```python
from build123d import *

# Parameters (mm, degrees)
BOSS_EXTRUDE1_DEPTH      = 5
BOSS_EXTRUDE2_DEPTH      = 4
SKETCH3_W                = 3
SKETCH3_H                = 52.6
BOSS_EXTRUDE3_DEPTH      = 7
SKETCH4_R                = 2.5
BOSS_EXTRUDE4_DEPTH      = 5.5
SKETCH5_R                = 3.7
CUT_EXTRUDE2_DEPTH       = 1.6
CUT_EXTRUDE4_DEPTH       = 1.6
SKETCH7_R                = 2.5
CUT_EXTRUDE6_DEPTH       = 1.6
SKETCH8_R                = 1.5
CUT_EXTRUDE8_DEPTH       = 4
M2_CLEARANCE_HOLE1_D     = 2.4
M2_CLEARANCE_HOLE1_DEPTH = 5
M2_CLEARANCE_HOLE1_TIP   = 0.721032743
M2_CLEARANCE_HOLE2_D     = 2.4
M2_CLEARANCE_HOLE2_DEPTH = 5
M2_CLEARANCE_HOLE2_TIP   = 0.721032743
M2_CLEARANCE_HOLE3_D     = 2.4
M2_CLEARANCE_HOLE3_DEPTH = 35
M2_CLEARANCE_HOLE4_D     = 2.4
M2_CLEARANCE_HOLE4_DEPTH = 35
M2_CLEARANCE_HOLE5_D     = 2.4
M2_CLEARANCE_HOLE5_DEPTH = 35
M2_CLEARANCE_HOLE6_D     = 2.4
M2_CLEARANCE_HOLE6_DEPTH = 35
FILLET1_R                = 2
SKETCH21_W               = 15
SKETCH21_H               = 7
CUT_EXTRUDE10_DEPTH      = 4
SKETCH22_W               = 8
SKETCH22_H               = 9
CUT_EXTRUDE11_DEPTH      = 2.5


with BuildPart() as part:
    # Sketch1 → Boss-Extrude1 (new body)
    with BuildSketch(Plane(origin=(0, 19.3, 0), x_dir=(1, 0, 0), z_dir=(0, 1, 0))):
        with BuildLine():
            Line((5.5, -7), (33.5, -7))
            Line((33.5, -7), (33.5, 7))
            Line((33.5, 7), (5.5, 7))
            ThreePointArc((5.5, 7), (-1.5, 0), (5.5, -7))
        make_face()
    extrude(amount=BOSS_EXTRUDE1_DEPTH)



with BuildPart() as body_2:
    # Sketch2 → Boss-Extrude2 (new body)
    with BuildSketch(Plane(origin=(0, -28.3, 0), x_dir=(1, 0, 0), z_dir=(0, 1, 0))):
        with BuildLine():
            Line((5.5, -7), (33.5, -7))
            Line((33.5, -7), (33.5, 7))
            Line((33.5, 7), (5.5, 7))
            ThreePointArc((5.5, 7), (-1.5, 0), (5.5, -7))
        make_face()
    extrude(amount=BOSS_EXTRUDE2_DEPTH)


with BuildPart() as part_1:
    add(part.part)

    add(body_2.part)  # Boss-Extrude3 merges body 2
    # Sketch3 → Boss-Extrude3 (add, symmetric)
    with BuildSketch(Plane.XY):
        with Locations((32, -2)):
            Rectangle(SKETCH3_W, SKETCH3_H)
    extrude(amount=BOSS_EXTRUDE3_DEPTH, both=True)

    # Sketch4 → Boss-Extrude4 (add)
    with BuildSketch(Plane(origin=(0, 24.3, 0), x_dir=(1, 0, 0), z_dir=(0, 1, 0))):
        with Locations(Location((5.5, 0, 0), (0, 0, 270))):
            Circle(SKETCH4_R)
    extrude(amount=BOSS_EXTRUDE4_DEPTH)

    # Sketch5 → Cut-Extrude2 (cut)
    with BuildSketch(Plane(origin=(0, 19.3, 0), x_dir=(1, 0, 0), z_dir=(0, 1, 0))):
        with Locations(Location((5.5, 0, 0), (0, 0, 270))):
            Circle(SKETCH5_R)
    extrude(amount=CUT_EXTRUDE2_DEPTH, mode=Mode.SUBTRACT)

    # Sketch6 → Cut-Extrude4 (cut)
    with BuildSketch(Plane(origin=(0, 19.3, 0), x_dir=(1, 0, 0), z_dir=(0, 1, 0))):
        with BuildLine():
            Line((5.5, -2.7), (20.7, -2.7))
            Line((20.7, -2.7), (20.7, 2.7))
            Line((20.7, 2.7), (5.5, 2.7))
            ThreePointArc((5.5, 2.7), (2.8, 0), (5.5, -2.7))
        make_face()
    extrude(amount=CUT_EXTRUDE4_DEPTH, mode=Mode.SUBTRACT)

    # Sketch7 → Cut-Extrude6 (cut)
    with BuildSketch(Plane(origin=(0, 20.9, 0), x_dir=(1, 0, 0), z_dir=(0, 1, 0))):
        with Locations(Location((5.5, 0, 0), (0, 0, 270))):
            Circle(SKETCH7_R)
    extrude(amount=CUT_EXTRUDE6_DEPTH, mode=Mode.SUBTRACT)

    # Sketch8 → Cut-Extrude8 (cut)
    with BuildSketch(Plane(origin=(0, -28.3, 0), x_dir=(1, 0, 0), z_dir=(0, 1, 0))):
        with Locations(Location((5.5, 0, 0), (0, 0, 270))):
            Circle(SKETCH8_R)
    extrude(amount=CUT_EXTRUDE8_DEPTH, mode=Mode.SUBTRACT)

    # M2 Clearance Hole1
    with Locations(Plane(origin=(0, 24.3, 0), x_dir=(1, 0, 0), z_dir=(0, 1, 0))):
        with Locations((15.5, 0)):
            Hole(M2_CLEARANCE_HOLE1_D / 2, depth=M2_CLEARANCE_HOLE1_DEPTH)
            with Locations((0, 0, -(M2_CLEARANCE_HOLE1_DEPTH + M2_CLEARANCE_HOLE1_TIP / 2))):  # 118° drill point
                Cone(0, M2_CLEARANCE_HOLE1_D / 2, M2_CLEARANCE_HOLE1_TIP, mode=Mode.SUBTRACT)

    # M2 Clearance Hole2
    with Locations(Plane(origin=(0, 24.3, 0), x_dir=(1, 0, 0), z_dir=(0, 1, 0))):
        with Locations((18.5, 0)):
            Hole(M2_CLEARANCE_HOLE2_D / 2, depth=M2_CLEARANCE_HOLE2_DEPTH)
            with Locations((0, 0, -(M2_CLEARANCE_HOLE2_DEPTH + M2_CLEARANCE_HOLE2_TIP / 2))):  # 118° drill point
                Cone(0, M2_CLEARANCE_HOLE2_D / 2, M2_CLEARANCE_HOLE2_TIP, mode=Mode.SUBTRACT)

    # M2 Clearance Hole3
    with Locations(Plane(origin=(33.5, 0, 0), x_dir=(0, 0, -1), z_dir=(1, 0, 0))):
        with Locations((4.5, -4.5)):
            Hole(M2_CLEARANCE_HOLE3_D / 2, depth=M2_CLEARANCE_HOLE3_DEPTH)

    # M2 Clearance Hole4
    with Locations(Plane(origin=(33.5, 0, 0), x_dir=(0, 0, -1), z_dir=(1, 0, 0))):
        with Locations((-4.5, -4.5)):
            Hole(M2_CLEARANCE_HOLE4_D / 2, depth=M2_CLEARANCE_HOLE4_DEPTH)

    # M2 Clearance Hole5
    with Locations(Plane(origin=(33.5, 0, 0), x_dir=(0, 0, -1), z_dir=(1, 0, 0))):
        with Locations((4.5, 4.5)):
            Hole(M2_CLEARANCE_HOLE5_D / 2, depth=M2_CLEARANCE_HOLE5_DEPTH)

    # M2 Clearance Hole6
    with Locations(Plane(origin=(33.5, 0, 0), x_dir=(0, 0, -1), z_dir=(1, 0, 0))):
        with Locations((-4.5, 4.5)):
            Hole(M2_CLEARANCE_HOLE6_D / 2, depth=M2_CLEARANCE_HOLE6_DEPTH)

    # Fillet1
    fillet1_edges = [part_1.edges().sort_by_distance(p)[0] for p in [
        (30.5, 19.3, 0),
        (30.5, -24.3, 0),
    ]]
    fillet(fillet1_edges, radius=FILLET1_R)

    # Sketch21 → Cut-Extrude10 (cut)
    with BuildSketch(Plane(origin=(0, -28.3, 0), x_dir=(1, 0, 0), z_dir=(0, 1, 0))):
        with Locations((19.5, 0)):
            Rectangle(SKETCH21_W, SKETCH21_H)
    extrude(amount=CUT_EXTRUDE10_DEPTH, mode=Mode.SUBTRACT)

    # Sketch22 → Cut-Extrude11 (cut)
    with BuildSketch(Plane(origin=(0, 24.3, 0), x_dir=(1, 0, 0), z_dir=(0, 1, 0))):
        with Locations((25, 0)):
            Rectangle(SKETCH22_W, SKETCH22_H)
    extrude(amount=-CUT_EXTRUDE11_DEPTH, mode=Mode.SUBTRACT)


solid = part_1.part
```
Source: CAD feature listing. Evaluate the final solid. Frame: model axes, mm. A direction names the side the tool comes from. Give positions to 0.01 mm unless a question says otherwise; leave off trailing zeros. Loops run counter-clockwise (first coordinate to the right, second up) from the corner with the lowest first, then second, coordinate; pieces in that order, holes last. Notation, with made-up numbers: (75.25, -32) -> (109.25, -32) arc R36 ccw to (109.25, 6) -> close; hole circle Ø1 at (-32.75, 53.5). An arc over 180 degrees is marked (long way). Put each result on its own line as item: value. Start each with the question number.
1) Cut plane B-B (y = -4.5). Return loops of the section in (x, z), then the cut area to 3 significant figures.
2) Draft query along X for faces 1 (the face through (1.8, 20.1, -0.1)), 2 (the face through (16, -28.3, 5)), 3 (the face through (29.9, -23.73, -0.1)). Return one class per face: released by +X, released by -X, zero draft, split by the parting line, or undercut.
3) Cut plane A-A (x = 10.5). Return loops of the section in (y, z).
4) Reachability of faces 4 (the face through (25, 21.8, 0)), 5 (the face through (17, 19.3, -3)), 6 (the face through (27, -26, 0)) from +Z, -Z, +X, -X, +Y, -Y: full face, straight path, thin tool, end or side. Return the list, or none.
5) Contact query for flat-ended pins moving along their axis: P1, Ø2.5, axis at x = 26, z = 1, coming from the +Y side; P2, Ø4, axis at x = 18.5, z = 3, coming from the +Y side; P3, Ø4, axis at y = 4.5, z = -4.5, coming from the -X side. Output: stop coordinate, or through.
6) Material intervals for probe 1 along Y at (x, z) = (31.5, -4.5); probe 2 along Z at (x, y) = (25.5, 24); probe 3 along Y at (x, z) = (28.5, -2.5), sorted ascending.
7) Cut plane C-C (x = 23.5). Return loops of the section in (y, z), then the cut area to 3 significant figures.
8) Cut plane D-D (x = 18.5). Return loops of the section in (y, z).
Results are:
1. outline: (30.5, -7) -> (33.5, -7) -> (33.5, -5.7) -> (30.5, -5.7) -> close; (30.5, -3.3) -> (33.5, -3.3) -> (33.5, 3.3) -> (30.5, 3.3) -> close; (30.5, 5.7) -> (33.5, 5.7) -> (33.5, 7) -> (30.5, 7) -> close
1. area: 27.6 mm2
2. face 1: undercut
2. face 2: zero draft
2. face 3: released by -X
3. outline: (-28.3, -7) -> (-24.3, -7) -> (-24.3, 7) -> (-28.3, 7) -> close; (19.3, -7) -> (24.3, -7) -> (24.3, 7) -> (19.3, 7) -> (19.3, 2.7) -> (20.9, 2.7) -> (20.9, -2.7) -> (19.3, -2.7) -> close
4. face 4: +Y
4. face 5: +Z, -Z, -X
4. face 6: -Y
5. P1: stops at y = 21.8
5. P2: stops at y = 24.3
5. P3: stops at x = 30.5
6. probe 1: y = -28.3 to -5.7, -3.3 to 3.3, 5.7 to 24.3
6. probe 2: z = -7 to -4.5, 4.5 to 7
6. probe 3: y = -28.3 to -24.3, 19.3 to 21.8
7. outline: (-28.3, -7) -> (-24.3, -7) -> (-24.3, -3.5) -> (-28.3, -3.5) -> close; (-28.3, 3.5) -> (-24.3, 3.5) -> (-24.3, 7) -> (-28.3, 7) -> close; (19.3, -7) -> (24.3, -7) -> (24.3, -4.5) -> (21.8, -4.5) -> (21.8, 4.5) -> (24.3, 4.5) -> (24.3, 7) -> (19.3, 7) -> close
7. area: 75.5 mm2
8. outline: (-28.3, -7) -> (-24.3, -7) -> (-24.3, -3.5) -> (-28.3, -3.5) -> close; (-28.3, 3.5) -> (-24.3, 3.5) -> (-24.3, 7) -> (-28.3, 7) -> close; (19.3, -7) -> (24.3, -7) -> (24.3, -1.2) -> (20.9, -1.2) -> (20.9, -2.7) -> (19.3, -2.7) -> close; (19.3, 2.7) -> (20.9, 2.7) -> (20.9, 1.2) -> (24.3, 1.2) -> (24.3, 7) -> (19.3, 7) -> close
